Build history of the part. All positions in model axes, mm. Face numbers are marked on the shaded views. A direction names the side the tool comes from. Round coordinates to 2 decimals unless told otherwise and drop trailing zeros. Write each loop counter-clockwise with the first axis right and the second up, starting at its lowest first coordinate (ties: lowest second). Pieces come first, ordered by that corner, then holes.
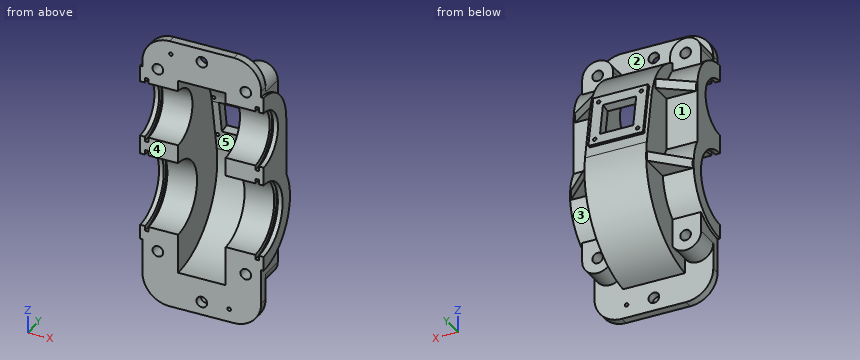
from build123d import *

# Parameters (mm, degrees)
EXTRUDE_1_DEPTH             = 7
EXTRUDE_2_DEPTH             = 52
EXTRUDE_START               = -26
EXTRUDE_4_DEPTH             = 52
SKETCH_4_R                  = 13
SKETCH_4_W                  = 26
SKETCH_4_H                  = 38
SKETCH_4_H_2                = 45
EXTRUDE_5_DEPTH             = 20
RIB_5_REACH                 = 188.625
SKETCH_5_WALL_W             = 406.05642967
SKETCH_5_WALL_H             = 8
RIB_6_REACH                 = 162.714
SKETCH_6_WALL_W             = 359.136664294
SKETCH_6_WALL_H             = 8
CUT_EXTRUDE_1_REACH         = 143.06
SKETCH_7_R                  = 4.5
CUT_EXTRUDE_2_REACH         = 135.334
SKETCH_8_R                  = 4.5
PATTERN_LINEAR_1_COUNT      = 2
PATTERN_LINEAR_1_PITCH      = 74
PATTERN_LINEAR_1_COUNT_DIR2 = 2
PATTERN_LINEAR_1_PITCH_DIR2 = 158
CUT_EXTRUDE_3_REACH         = 143.06
SKETCH_9_R                  = 1.5
CUT_EXTRUDE_4_REACH         = 143.06
SKETCH_10_R                 = 1.5
SKETCH_11_R                 = 23.5
SKETCH_11_R_2               = 31
CUT_EXTRUDE_5_DEPTH         = 285.5
CUT_EXTRUDE_START           = 48
SKETCH_13_R                 = 27.5
SKETCH_13_R_2               = 35
CUT_EXTRUDE_6_DEPTH         = 3
CUT_EXTRUDE_7_DEPTH         = 20
EXTRUDE_6_DEPTH             = 23
CUT_EXTRUDE_8_REACH         = 154.782
SKETCH_17_W                 = 28
SKETCH_17_H                 = 28
CUT_EXTRUDE_9_REACH         = 154.782
SKETCH_18_R                 = 1.5


# Read off the part's stored shape, not the designer's step: the extrude step
with BuildPart() as part:
    # Sketch 1 → Extrude 1 (new body)
    with BuildSketch(Plane(origin=(0, 0, 0), x_dir=(1, 0, 0), z_dir=(0, 1, 0))):
        with BuildLine():
            Line((-27, 115), (27, 115))
            ThreePointArc((27, 115), (43.263455967, 108.263455967), (50, 92))
            Line((50, 92), (50, -92))
            ThreePointArc((50, -92), (43.263455967, -108.263455967), (27, -115))
            Line((27, -115), (-27, -115))
            ThreePointArc((-27, -115), (-43.263455967, -108.263455967), (-50, -92))
            Line((-50, -92), (-50, 92))
            ThreePointArc((-50, 92), (-43.263455967, 108.263455967), (-27, 115))
        make_face()
    extrude(amount=EXTRUDE_1_DEPTH)

    # Sketch 2 → Extrude 2 (add, symmetric)
    with BuildSketch(Plane(origin=(0, 0, 0), x_dir=(0, 0, -1), z_dir=(1, 0, 0))):
        with BuildLine():
            ThreePointArc((63, 0), (41.294567395, 37.356945799), (-1.9089023, 37))
            ThreePointArc((-1.9089023, 37), (-11.440919182, 29.33374509), (-18.428571429, 19.293649161))
            ThreePointArc((-18.428571429, 19.293649161), (-14.382989618, 10.021405661), (-13, 0))
            Line((-13, 0), (63, 0))
        make_face()
        with BuildLine():
            ThreePointArc((-18.428571429, 19.293649161), (-31.901174333, 32.271233467), (-50, 37))
            ThreePointArc((-50, 37), (-76.162950904, 26.162950904), (-87, 0))
            Line((-87, 0), (-23, 0))
            ThreePointArc((-23, 0), (-21.841537803, 9.913915185), (-18.428571429, 19.293649161))
        make_face()
        with BuildLine():
            Line((-1.9089023, 37), (-50, 37))
            ThreePointArc((-50, 37), (-31.901174333, 32.271233467), (-18.428571429, 19.293649161))
            ThreePointArc((-18.428571429, 19.293649161), (-11.440919182, 29.33374509), (-1.9089023, 37))
        make_face()
        with BuildLine():
            ThreePointArc((-13, 0), (-14.382989618, 10.021405661), (-18.428571429, 19.293649161))
            ThreePointArc((-18.428571429, 19.293649161), (-21.841537803, 9.913915185), (-23, 0))
            Line((-23, 0), (-13, 0))
        make_face()
    extrude(amount=EXTRUDE_2_DEPTH, both=True)

    # Extrude 4 outline → Extrude 4 (add)
    with BuildSketch(Plane(origin=(0, 0, 0), x_dir=(0, 0, -1), z_dir=(1, 0, 0)).offset(EXTRUDE_START)):
        with BuildLine():
            ThreePointArc((-37.166666667, 61.075545206), (-71.630787409, 42.511316468), (-88.103571325, 7))
            Line((-88.103571325, 7), (-86.331804249, 7))
            ThreePointArc((-86.331804249, 7), (-73.558437979, 28.530685235), (-50, 37))
            Line((-50, 37), (-1.9089023, 37))
            ThreePointArc((-1.9089023, 37), (38.172561692, 38.97124583), (62.426406871, 7))
            Line((62.426406871, 7), (89.649120597, 7))
            ThreePointArc((89.649120597, 7), (62.299651693, 55.774003502), (7.956989247, 68.956260717))
            Line((7.956989247, 68.956260717), (-37.166666667, 61.075545206))
        make_face()
    extrude(amount=EXTRUDE_4_DEPTH)

    # Sketch 4 → Extrude 5 (add)
    with BuildSketch(Plane(origin=(0, 7, 0), x_dir=(1, 0, 0), z_dir=(0, 1, 0))):
        with Locations((37, -88)):
            Circle(SKETCH_4_R)
        with Locations((-37, -88)):
            Circle(SKETCH_4_R)
        with Locations((37, 70)):
            Circle(SKETCH_4_R)
        with Locations((-37, 70)):
            Circle(SKETCH_4_R)
        with Locations((37, -69)):
            Rectangle(SKETCH_4_W, SKETCH_4_H)
        with Locations((-37, -69)):
            Rectangle(SKETCH_4_W, SKETCH_4_H)
        with Locations((37, 47.5)):
            Rectangle(SKETCH_4_W, SKETCH_4_H_2)
        with Locations((-37, 47.5)):
            Rectangle(SKETCH_4_W, SKETCH_4_H_2)
    extrude(amount=EXTRUDE_5_DEPTH)

    # Sketch 5 wall → Rib 5 (add, up to next)
    with BuildSketch(Plane(origin=(38.5, 46, 50), x_dir=(-0.811534341451, 0.584304725845, 0), z_dir=(-0.584304725845, -0.811534341451, 0)), mode=Mode.PRIVATE) as rib_5_sk1:
        Rectangle(SKETCH_5_WALL_W, SKETCH_5_WALL_H)
    rib_5_tool1 = extrude(rib_5_sk1.sketch, amount=RIB_5_REACH, mode=Mode.PRIVATE) - part.part
    rib_5 = rib_5_tool1.solids().sort_by_distance((38.5, 46, 50))[0]
    add(rib_5)

    # Mirror 1: Rib 5 across plane
    add(rib_5.mirror(Plane(origin=(0, 0, 0), x_dir=(0, 0, 1), z_dir=(1, 0, 0))))

    # Sketch 6 wall → Rib 6 (add, up to next)
    with BuildSketch(Plane(origin=(38.590481041, 55.659219169, -20), x_dir=(-0.705179186997, 0.709029134963, 0), z_dir=(-0.709029134963, -0.705179186997, 0)), mode=Mode.PRIVATE) as rib_6_sk1:
        Rectangle(SKETCH_6_WALL_W, SKETCH_6_WALL_H)
    rib_6_tool1 = extrude(rib_6_sk1.sketch, amount=RIB_6_REACH, mode=Mode.PRIVATE) - part.part
    rib_6 = rib_6_tool1.solids().sort_by_distance((38.590481041, 55.659219169, -20))[0]
    add(rib_6)

    # Mirror 2: Rib 6 across plane
    add(rib_6.mirror(Plane(origin=(0, 0, 0), x_dir=(0, 0, 1), z_dir=(1, 0, 0))))

    # Sketch 7 → Cut-Extrude 1 (cut, up to next)
    with BuildSketch(Plane(origin=(0, 7, 0), x_dir=(1, 0, 0), z_dir=(0, 1, 0)), mode=Mode.PRIVATE) as cut_extrude_1_sk1:
        with Locations(Location((0, 104, 0), (0, 0, 270))):
            Circle(SKETCH_7_R)
    cut_extrude_1_tool1 = extrude(cut_extrude_1_sk1.sketch, amount=-CUT_EXTRUDE_1_REACH, mode=Mode.PRIVATE) & part.part
    # Sketch 7 → Cut-Extrude 1 (cut, up to next)
    with BuildSketch(Plane(origin=(0, 7, 0), x_dir=(1, 0, 0), z_dir=(0, 1, 0)), mode=Mode.PRIVATE) as cut_extrude_1_sk2:
        with Locations(Location((0, -104, 0), (0, 0, 270))):
            Circle(SKETCH_7_R)
    cut_extrude_1_tool2 = extrude(cut_extrude_1_sk2.sketch, amount=-CUT_EXTRUDE_1_REACH, mode=Mode.PRIVATE) & part.part
    add(cut_extrude_1_tool1.solids().sort_by_distance((0, 7, -104))[0], mode=Mode.SUBTRACT)
    add(cut_extrude_1_tool2.solids().sort_by_distance((0, 7, 104))[0], mode=Mode.SUBTRACT)

    # Sketch 8 → Cut-Extrude 2 (cut, up to next)
    with BuildSketch(Plane(origin=(0, 27, 0), x_dir=(1, 0, 0), z_dir=(0, 1, 0)), mode=Mode.PRIVATE) as cut_extrude_2_sk1:
        with Locations(Location((-37, 70, 0), (0, 0, 270))):
            Circle(SKETCH_8_R)
    cut_extrude_2_tool1 = extrude(cut_extrude_2_sk1.sketch, amount=-CUT_EXTRUDE_2_REACH, mode=Mode.PRIVATE) & part.part
    cut_extrude_2 = cut_extrude_2_tool1.solids().sort_by_distance((-37, 27, -70))[0]
    add(cut_extrude_2, mode=Mode.SUBTRACT)

    # Pattern Linear 1: Cut-Extrude 2 2 × 2
    with Locations(*[(i * PATTERN_LINEAR_1_PITCH, 0, j * PATTERN_LINEAR_1_PITCH_DIR2) for i in range(PATTERN_LINEAR_1_COUNT) for j in range(PATTERN_LINEAR_1_COUNT_DIR2) if (i, j) != (0, 0)]):
        add(cut_extrude_2, mode=Mode.SUBTRACT)

    # Sketch 9 → Cut-Extrude 3 (cut, up to next)
    with BuildSketch(Plane(origin=(0, 7, 0), x_dir=(1, 0, 0), z_dir=(0, 1, 0)), mode=Mode.PRIVATE) as cut_extrude_3_sk1:
        with Locations(Location((-26, -104, 0), (0, 0, 270))):
            Circle(SKETCH_9_R)
    cut_extrude_3_tool1 = extrude(cut_extrude_3_sk1.sketch, amount=-CUT_EXTRUDE_3_REACH, mode=Mode.PRIVATE) & part.part
    add(cut_extrude_3_tool1.solids().sort_by_distance((-26, 7, 104))[0], mode=Mode.SUBTRACT)

    # Sketch 10 → Cut-Extrude 4 (cut, up to next)
    with BuildSketch(Plane(origin=(0, 7, 0), x_dir=(1, 0, 0), z_dir=(0, 1, 0)), mode=Mode.PRIVATE) as cut_extrude_4_sk1:
        with Locations(Location((23, 104, 0), (0, 0, 270))):
            Circle(SKETCH_10_R)
    cut_extrude_4_tool1 = extrude(cut_extrude_4_sk1.sketch, amount=-CUT_EXTRUDE_4_REACH, mode=Mode.PRIVATE) & part.part
    add(cut_extrude_4_tool1.solids().sort_by_distance((23, 7, -104))[0], mode=Mode.SUBTRACT)

    # Sketch 11 → Cut-Extrude 5 (cut, symmetric)
    with BuildSketch(Plane(origin=(0, 0, 0), x_dir=(0, 0, -1), z_dir=(1, 0, 0))):
        with Locations((-50, 0)):
            Circle(SKETCH_11_R)
        with Locations((20, 0)):
            Circle(SKETCH_11_R_2)
    extrude(amount=CUT_EXTRUDE_5_DEPTH, both=True, mode=Mode.SUBTRACT)

    # Sketch 13 → Cut-Extrude 6 (cut)
    with BuildSketch(Plane(origin=(0, 0, 0), x_dir=(0, 0, -1), z_dir=(1, 0, 0)).offset(CUT_EXTRUDE_START)):
        with Locations((-50, 0)):
            Circle(SKETCH_13_R)
        with Locations((20, 0)):
            Circle(SKETCH_13_R_2)
    cut_extrude_6 = extrude(amount=-CUT_EXTRUDE_6_DEPTH, mode=Mode.SUBTRACT)

    # Mirror 3: Cut-Extrude 6 across plane
    add(cut_extrude_6.mirror(Plane(origin=(0, 0, 0), x_dir=(0, 0, 1), z_dir=(1, 0, 0))), mode=Mode.SUBTRACT)

    # Sketch 15 → Cut-Extrude 7 (cut, symmetric)
    with BuildSketch(Plane(origin=(0, 0, 0), x_dir=(0, 0, -1), z_dir=(1, 0, 0))):
        with BuildLine():
            Line((-82.5, 0), (84, 0))
            ThreePointArc((84, 0), (61.178342778, 48.993306543), (8.989247312, 63.045724084))
            Line((8.989247312, 63.045724084), (-36.134408602, 55.165008573))
            ThreePointArc((-36.134408602, 55.165008573), (-69.369143225, 36.031049931), (-82.5, 0))
        make_face()
    extrude(amount=CUT_EXTRUDE_7_DEPTH, both=True, mode=Mode.SUBTRACT)

    # Sketch 16 → Extrude 6 (add, symmetric)
    with BuildSketch(Plane(origin=(0, 0, 0), x_dir=(0, 0, -1), z_dir=(1, 0, 0))):
        Polygon((-46.682604529, 61.443886786), (-45.822389476, 56.518439592), (-0.508275291, 64.432418086), (-1.368490344, 69.35786528), align=None)
    extrude(amount=EXTRUDE_6_DEPTH, both=True)

    # Sketch 17 → Cut-Extrude 8 (cut, up to next)
    with BuildSketch(Plane(origin=(0, 67.536884536, 11.795120823), x_dir=(1, 0, 0), z_dir=(0, 0.9850894388080457, 0.17204301075268907)), mode=Mode.PRIVATE) as cut_extrude_8_sk1:
        with Locations((0, -12.415549423)):
            Rectangle(SKETCH_17_W, SKETCH_17_H)
    cut_extrude_8_tool1 = extrude(cut_extrude_8_sk1.sketch, amount=-CUT_EXTRUDE_8_REACH, mode=Mode.PRIVATE) & part.part
    add(cut_extrude_8_tool1.solids().sort_by_distance((0, 65.400876, 24.025547))[0], mode=Mode.SUBTRACT)

    # Sketch 18 → Cut-Extrude 9 (cut, up to next)
    with BuildSketch(Plane(origin=(0, 67.536884536, 11.795120823), x_dir=(1, 0, 0), z_dir=(0, 0.9850894388080457, 0.17204301075268907)), mode=Mode.PRIVATE) as cut_extrude_9_sk1:
        with Locations(Location((-18, -30.415549423, 0), (0, 0, 270))):
            Circle(SKETCH_18_R)
    cut_extrude_9_tool1 = extrude(cut_extrude_9_sk1.sketch, amount=-CUT_EXTRUDE_9_REACH, mode=Mode.PRIVATE) & part.part
    # Sketch 18 → Cut-Extrude 9 (cut, up to next)
    with BuildSketch(Plane(origin=(0, 67.536884536, 11.795120823), x_dir=(1, 0, 0), z_dir=(0, 0.9850894388080457, 0.17204301075268907)), mode=Mode.PRIVATE) as cut_extrude_9_sk2:
        with Locations(Location((18, -30.415549423, 0), (0, 0, 270))):
            Circle(SKETCH_18_R)
    cut_extrude_9_tool2 = extrude(cut_extrude_9_sk2.sketch, amount=-CUT_EXTRUDE_9_REACH, mode=Mode.PRIVATE) & part.part
    # Sketch 18 → Cut-Extrude 9 (cut, up to next)
    with BuildSketch(Plane(origin=(0, 67.536884536, 11.795120823), x_dir=(1, 0, 0), z_dir=(0, 0.9850894388080457, 0.17204301075268907)), mode=Mode.PRIVATE) as cut_extrude_9_sk3:
        with Locations(Location((-18, 5.584450577, 0), (0, 0, 270))):
            Circle(SKETCH_18_R)
    cut_extrude_9_tool3 = extrude(cut_extrude_9_sk3.sketch, amount=-CUT_EXTRUDE_9_REACH, mode=Mode.PRIVATE) & part.part
    # Sketch 18 → Cut-Extrude 9 (cut, up to next)
    with BuildSketch(Plane(origin=(0, 67.536884536, 11.795120823), x_dir=(1, 0, 0), z_dir=(0, 0.9850894388080457, 0.17204301075268907)), mode=Mode.PRIVATE) as cut_extrude_9_sk4:
        with Locations(Location((18, 5.584450577, 0), (0, 0, 270))):
            Circle(SKETCH_18_R)
    cut_extrude_9_tool4 = extrude(cut_extrude_9_sk4.sketch, amount=-CUT_EXTRUDE_9_REACH, mode=Mode.PRIVATE) & part.part
    add(cut_extrude_9_tool1.solids().sort_by_distance((-18, 62.304102, 41.757157))[0], mode=Mode.SUBTRACT)
    add(cut_extrude_9_tool2.solids().sort_by_distance((18, 62.304102, 41.757157))[0], mode=Mode.SUBTRACT)
    add(cut_extrude_9_tool3.solids().sort_by_distance((-18, 68.49765, 6.293938))[0], mode=Mode.SUBTRACT)
    add(cut_extrude_9_tool4.solids().sort_by_distance((18, 68.49765, 6.293938))[0], mode=Mode.SUBTRACT)


solid = part.part
1) Slice it at A-A (x = -11.5). Write the cut outline in (y, z), plus the area to 3 significant figures.
Results:
outline: (0, -115) - (7, -115) - (7, -89.65) arc R70 ccw to (68.96, -7.96) - (67.39, 1.02) - (69.36, 1.37) - (67.81, 10.23) - (59.93, 8.86) - (63.05, -8.99) arc R64 cw to (0, -84) - close; (0, 82.5) arc R56 cw to (55.11, 36.44) - (62.99, 37.82) - (61.44, 46.68) - (58.78, 46.22) arc R62 ccw to (7, 88.1) - (7, 115) - (0, 115) - close
area: 1,700 mm2
2) Mould opens along Z. For the marked faces 4 and 5 say: released by +Z, released by -Z, zero draft, split by the parting line, or undercut.
Results:
face 4: zero draft
face 5: undercut
3) Pin check, flat tips, straight feed: pin 1 Ø1 at (x, z) = (-2.5, -74) entering from -Y; pin 2 Ø6 at (x, z) = (-15, 79.5) entering from +Y; pin 3 Ø4 at (x, y) = (-11.5, 29) entering from -Z. Stop position of each tip, or through.
Results:
pin 1: stops at y = 33.55
pin 2: stops at y = 36.66
pin 3: stops at z = -84.58
4) Which spindle directions (+Z, -Z, +X, -X, +Y, -Y) get a long thin tool onto all of the face, cutting with end or side? Do the marked faces 1, 2 and 3. Say none if no direction does.
Results:
face 1: -X, +Y
face 2: +Z, +Y
face 3: +X, +Y
5) Slice it at B-B (x = 0). Write the cut outline in (y, z).
Results:
outline: (0, -115) - (7, -115) - (7, -108.5) - (0, -108.5) - close; (0, -99.5) - (7, -99.5) - (7, -89.65) arc R70 ccw to (68.96, -7.96) - (67.39, 1.02) - (69.36, 1.37) - (67.81, 10.23) - (59.93, 8.86) - (63.05, -8.99) arc R64 cw to (0, -84) - close; (0, 82.5) arc R56 cw to (55.11, 36.44) - (62.99, 37.82) - (61.44, 46.68) - (58.78, 46.22) arc R62 ccw to (7, 88.1) - (7, 99.5) - (0, 99.5) - close; (0, 108.5) - (7, 108.5) - (7, 115) - (0, 115) - close
6) Slice it at D-D (z = -32.5). Write the cut outline in (x, y).
Results:
outline: (-52, 28.37) - (-48, 28.37) - (-48, 32.69) - (-45, 32.69) - (-45, 28.37) - (-20, 28.37) - (-20, 62.77) - (20, 62.77) - (20, 28.37) - (45, 28.37) - (45, 32.69) - (48, 32.69) - (48, 28.37) - (52, 28.37) - (52, 41.14) - (26, 41.14) - (26, 68.87) - (-26, 68.87) - (-26, 41.14) - (-52, 41.14) - close
7) Wall check: L1, parallel to X at y = 11.5, z = -70; L2, parallel to X at y = 21.25, z = 88; L3, parallel to X at y = 2.5, z = -104. Give the ranges that are in metal, low to high.
Results:
L1: x = -50 to -41.5, -32.5 to -20, 20 to 32.5, 41.5 to 50
L2: x = -50 to -41.5, -32.5 to -24, 24 to 32.5, 41.5 to 50
L3: x = -46.62 to -4.5, 4.5 to 21.5, 24.5 to 46.62
8) Slice it at C-C (z = -87). Write the cut outline in (x, y), plus the area to 3 significant figures.
Results:
outline: (-50, 0) - (50, 0) - (50, 7) - (26, 7) - (26, 20.27) - (-26, 20.27) - (-26, 7) - (-50, 7) - close
area: 1,390 mm2
